from build123d import *

# Parameters (mm, degrees)
F0_W     = 130
F0_H     = 75
F1_DEPTH = 12
F3_DEPTH = 280
F5_W     = 75
F5_H     = 55
F6_DEPTH = 12
F7_D     = 12
F9_D     = 12
F9_DEPTH = 12
F9_TIP   = 3.6051637142


with BuildPart() as f1:
    # F0 (on Top) → F1 (new body)
    with BuildSketch(Plane.XY):
        Rectangle(F0_W, F0_H)
    extrude(amount=-F1_DEPTH)

    # F2 (on face) → F3 (join)
    with BuildSketch(Plane.XY):
        with BuildLine():
            Line((-19.05, -25.4), (19.05, -25.4))
            ThreePointArc((19.05, -25.4), (23.5401280605, -23.5401280605), (25.4, -19.05))
            Line((25.4, -19.05), (25.4, 19.05))
            ThreePointArc((25.4, 19.05), (23.5401280605, 23.5401280605), (19.05, 25.4))
            Line((19.05, 25.4), (-19.05, 25.4))
            ThreePointArc((-19.05, 25.4), (-23.5401280605, 23.5401280605), (-25.4, 19.05))
            Line((-25.4, 19.05), (-25.4, -19.05))
            ThreePointArc((-25.4, -19.05), (-23.5401280605, -23.5401280605), (-19.05, -25.4))
        make_face()
        with BuildLine():
            Line((-12.7, 19.05), (12.7, 19.05))
            ThreePointArc((12.7, 19.05), (17.1901280605, 17.1901280605), (19.05, 12.7))
            Line((19.05, 12.7), (19.05, -12.7))
            ThreePointArc((19.05, -12.7), (17.1901280605, -17.1901280605), (12.7, -19.05))
            Line((12.7, -19.05), (-12.7, -19.05))
            ThreePointArc((-12.7, -19.05), (-17.1901280605, -17.1901280605), (-19.05, -12.7))
            Line((-19.05, -12.7), (-19.05, 12.7))
            ThreePointArc((-19.05, 12.7), (-17.1901280605, 17.1901280605), (-12.7, 19.05))
        make_face(mode=Mode.SUBTRACT)
    extrude(amount=F3_DEPTH)

    # F5 (on face) → F6 (join)
    with BuildSketch(Plane.XY.offset(280)):
        Rectangle(F5_W, F5_H)
        with BuildLine():
            Line((19.05, -25.4), (-19.05, -25.4))
            ThreePointArc((-19.05, -25.4), (-23.5401280605, -23.5401280605), (-25.4, -19.05))
            Line((-25.4, -19.05), (-25.4, 19.05))
            ThreePointArc((-25.4, 19.05), (-23.5401280605, 23.5401280605), (-19.05, 25.4))
            Line((-19.05, 25.4), (19.05, 25.4))
            ThreePointArc((19.05, 25.4), (23.5401280605, 23.5401280605), (25.4, 19.05))
            Line((25.4, 19.05), (25.4, -19.05))
            ThreePointArc((25.4, -19.05), (23.5401280605, -23.5401280605), (19.05, -25.4))
        make_face(mode=Mode.SUBTRACT)
        with BuildLine():
            ThreePointArc((-25.4, -19.05), (-23.5401280605, -23.5401280605), (-19.05, -25.4))
            Line((-19.05, -25.4), (19.05, -25.4))
            ThreePointArc((19.05, -25.4), (23.5401280605, -23.5401280605), (25.4, -19.05))
            Line((25.4, -19.05), (25.4, 19.05))
            ThreePointArc((25.4, 19.05), (23.5401280605, 23.5401280605), (19.05, 25.4))
            Line((19.05, 25.4), (-19.05, 25.4))
            ThreePointArc((-19.05, 25.4), (-23.5401280605, 23.5401280605), (-25.4, 19.05))
            Line((-25.4, 19.05), (-25.4, -19.05))
        make_face()
        with BuildLine():
            Line((-19.05, -12.7), (-19.05, 12.7))
            ThreePointArc((-19.05, 12.7), (-17.1901280605, 17.1901280605), (-12.7, 19.05))
            Line((-12.7, 19.05), (12.7, 19.05))
            ThreePointArc((12.7, 19.05), (17.1901280605, 17.1901280605), (19.05, 12.7))
            Line((19.05, 12.7), (19.05, -12.7))
            ThreePointArc((19.05, -12.7), (17.1901280605, -17.1901280605), (12.7, -19.05))
            Line((12.7, -19.05), (-12.7, -19.05))
            ThreePointArc((-12.7, -19.05), (-17.1901280605, -17.1901280605), (-19.05, -12.7))
        make_face(mode=Mode.SUBTRACT)
        with BuildLine():
            ThreePointArc((-12.7, 19.05), (-17.1901280605, 17.1901280605), (-19.05, 12.7))
            Line((-19.05, 12.7), (-19.05, -12.7))
            ThreePointArc((-19.05, -12.7), (-17.1901280605, -17.1901280605), (-12.7, -19.05))
            Line((-12.7, -19.05), (12.7, -19.05))
            ThreePointArc((12.7, -19.05), (17.1901280605, -17.1901280605), (19.05, -12.7))
            Line((19.05, -12.7), (19.05, 12.7))
            ThreePointArc((19.05, 12.7), (17.1901280605, 17.1901280605), (12.7, 19.05))
            Line((12.7, 19.05), (-12.7, 19.05))
        make_face()
    extrude(amount=F6_DEPTH)

    # F7 (through all)
    with Locations(Plane.XY):
        with Locations((-53, 22.5), (53, 22.5), (53, -22.5), (-53, -22.5)):
            Hole(F7_D / 2)

    # F9
    with Locations(Plane.XY.offset(292)):
        with Locations((-22.5, -12.5), (22.5, -12.5)):
            Hole(F9_D / 2, depth=F9_DEPTH)
            with Locations((0, 0, -(F9_DEPTH + F9_TIP / 2))):  # 118° drill point
                Cone(0, F9_D / 2, F9_TIP, mode=Mode.SUBTRACT)


solid = f1.part
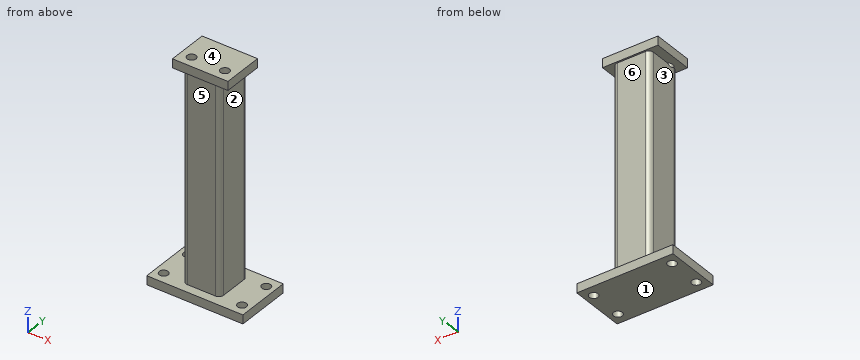
Geometry check sheet. Reference: the model listing, model coordinates, mm. Face numbers are marked on the shaded views. A direction names the side the tool comes from. Give positions to 0.01 mm unless a question says otherwise; leave off trailing zeros. Loops run counter-clockwise (first coordinate to the right, second up) from the corner with the lowest first, then second, coordinate; pieces in that order, holes last. Notation, with made-up numbers: M 11.25,10 L 69.25,10 A16 ccw 69.25,16 Z; hole C 51.25,86 d8. An arc over 180 degrees is marked long. Answer as a JSON object with one key per item and string values. Group by question number.
Item 1: Access from +Z, -Z, +X, -X, +Y, -Y to the whole of each face (thin tool, end or side, straight path). Record for the marked faces 5 and 6.
Item 2: Sectioned sample at D-D on x = -8. Record the boundary of the cut face in (y, z).
Item 3: Sectioned sample at C-C on y = -22.5. Record the boundary of the cut face in (x, z).
Item 4: Sectioned sample at B-B on z = 107. Record the boundary of the cut face in (x, y), plus the area to 3 significant figures.
Item 5: Gauge pin test, flat ends, axial feed: pin 1 (7 mm diameter, centred on x = 22.5, y = -12.5, fed in from +Z); pin 2 (5 mm diameter, centred on x = -3, z = 218, fed in from -Y); pin 3 (14 mm diameter, centred on x = 53, y = 22.5, fed in from -Z); pin 4 (11 mm diameter, centred on x = 53, y = -22.5, fed in from +Z). Record the tip position at first contact, or that the pin passes through.
Item 6: Material ranges on L1, parallel to X at y = 22, z = -4; L2, parallel to Z at x = -12, y = -17; L3, parallel to Y at x = 3, z = 140, recorded low to high.
Item 7: Sectioned sample at A-A on x = 53. Record the boundary of the cut face in (y, z).
Item 8: Mould release check, pull along Z, two halves, no side actions. Record for the marked faces 1, 2, 3 and 4: pulls with the +Z half, pulls with the -Z half, needs draft (parallel to the pull), parting line crosses it, or undercut.
Findings below:
{
 "1": {"face 5": "+X, -X, -Y", "face 6": "+X, -X, +Y"},
 "2": {"outline": "M -37.5,-12 L 37.5,-12 L 37.5,0 L 25.4,0 L 25.4,280 L 27.5,280 L 27.5,292 L -27.5,292 L -27.5,280 L -25.4,280 L -25.4,0 L -37.5,0 Z; hole M -19.05,0 L 19.05,0 L 19.05,280 L -19.05,280 Z"},
 "3": {"outline": "M -65,-12 L -59,-12 L -59,0 L -65,0 Z; M -47,-12 L 47,-12 L 47,0 L 24.38,0 L 24.38,280 L 37.5,280 L 37.5,292 L -37.5,292 L -37.5,280 L -24.38,280 L -24.38,0 L -47,0 Z; M 59,-12 L 65,-12 L 65,0 L 59,0 Z"},
 "4": {"outline": "M -25.4,-19.05 A6.35 ccw -19.05,-25.4 L 19.05,-25.4 A6.35 ccw 25.4,-19.05 L 25.4,19.05 A6.35 ccw 19.05,25.4 L -19.05,25.4 A6.35 ccw -25.4,19.05 Z; hole M -19.05,-12.7 A6.35 ccw -12.7,-19.05 L 12.7,-19.05 A6.35 ccw 19.05,-12.7 L 19.05,12.7 A6.35 ccw 12.7,19.05 L -12.7,19.05 A6.35 ccw -19.05,12.7 Z", "area": "1,130 mm2"},
 "5": {"pin 1": "z = 278.5", "pin 2": "y = -25.4", "pin 3": "z = -12", "pin 4": "through"},
 "6": {"L1": "-65 to -58.98, -47.02 to 47.02, 58.98 to 65", "L2": "-12 to 0, 280 to 292", "L3": "-25.4 to -19.05, 19.05 to 25.4"},
 "7": {"outline": "M -37.5,-12 L -28.5,-12 L -28.5,0 L -37.5,0 Z; M -16.5,-12 L 16.5,-12 L 16.5,0 L -16.5,0 Z; M 28.5,-12 L 37.5,-12 L 37.5,0 L 28.5,0 Z"},
 "8": {"face 1": "pulls with the -Z half", "face 2": "undercut", "face 3": "undercut", "face 4": "pulls with the +Z half"}
}
